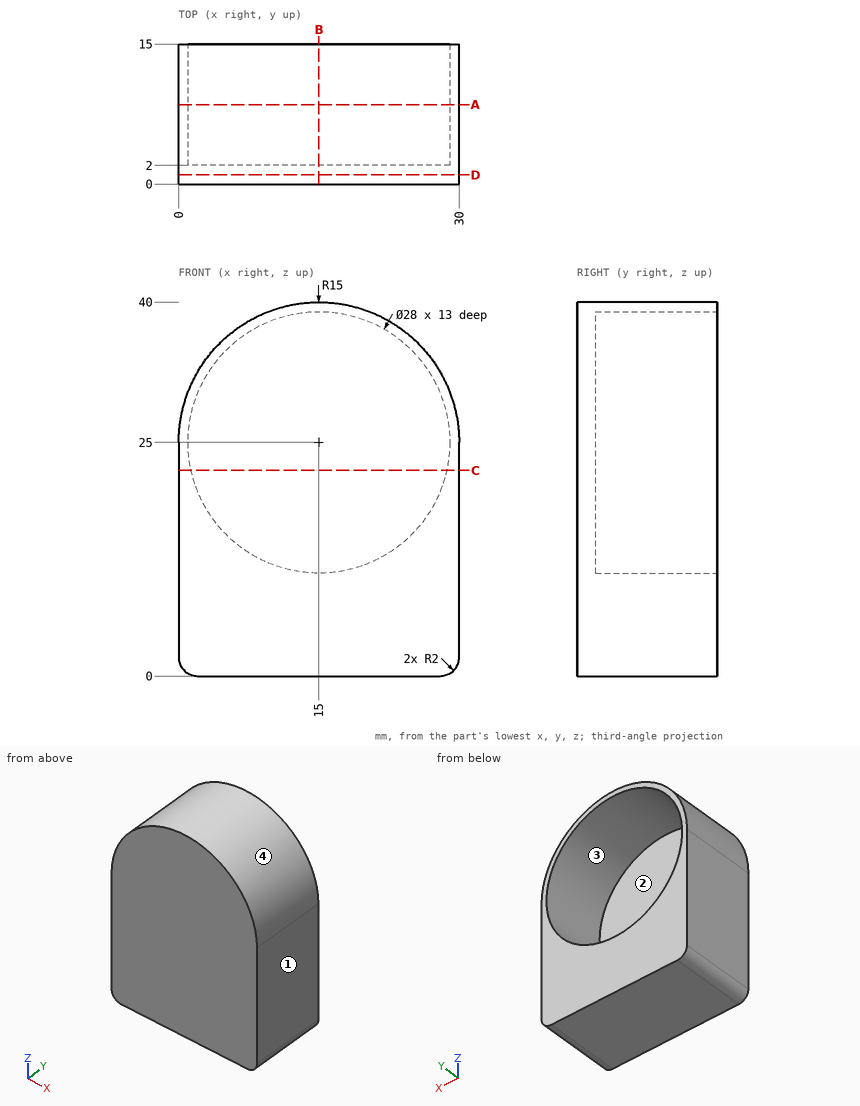
Answer from the drawing. Dimensions are ordinates in mm from the lowest x, y and z of the part. Round coordinates to 2 decimals unless told otherwise and drop trailing zeros. Loops run counter-clockwise (first coordinate to the right, second up) from the corner with the lowest first, then second, coordinate; pieces in that order, holes last.
Q1. Section C-C on z = 22 is taken. Write down the section's boundary in (x, y).
Q2. Section D-D on y = 1 is taken. Write down the section's boundary in (x, z).
Q3. Each of these flat-tipped pins is pushed along its axis until it touches: pin 1 (1.5 mm diameter, centred on y = 13, z = 28.5, fed in from +X); pin 2 (1.5 mm diameter, centred on x = 18, y = 8.5, fed in from +Z); pin 3 (5 mm diameter, centred on x = 19, y = 10, fed in from +Z). Where does it stop, or does it pass through?
Q4. Determine the mould class of the marked faces 1, 2, 3 and 4 for opening direction Z: released by +Z, released by -Z, zero draft, split by the parting line, or undercut.
Q5. Section A-A on y = 8.5 is taken. Write down the section's boundary in (x, z), and give its area (3 significant figures).
Q6. Consider probe 1 along Z at (x, y) = (15, 8.25); probe 2 along X at (y, z) = (9.5, 25); probe 3 along X at (y, z) = (11.75, 14). Determine where each line is inside the solid, lowest interval first.
Q7. Section B-B on x = 15 is taken. Write down the section's boundary in (y, z).
Output:
1. outline: (0, 0) - (30, 0) - (30, 15) - (28.67, 15) - (28.67, 2) - (1.33, 2) - (1.33, 15) - (0, 15) - close
2. outline: (0, 2) arc R2 ccw to (2, 0) - (28, 0) arc R2 ccw to (30, 2) - (30, 25) arc R15 ccw to (0, 25) - close
3. pin 1: stops at x = 29.75
3. pin 2: stops at z = 39.83
3. pin 3: stops at z = 39.92
4. face 1: zero draft
4. face 2: undercut
4. face 3: undercut
4. face 4: released by +Z
5. outline: (0, 2) arc R2 ccw to (2, 0) - (28, 0) arc R2 ccw to (30, 2) - (30, 25) arc R15 ccw to (0, 25) - close; hole circle Ø28 at (15, 25)
5. area: 486 mm2
6. probe 1: z = 0 to 11, 39 to 40
6. probe 2: x = 0 to 1, 29 to 30
6. probe 3: x = 0 to 6.34, 23.66 to 30
7. outline: (0, 0) - (15, 0) - (15, 11) - (2, 11) - (2, 39) - (15, 39) - (15, 40) - (0, 40) - close
